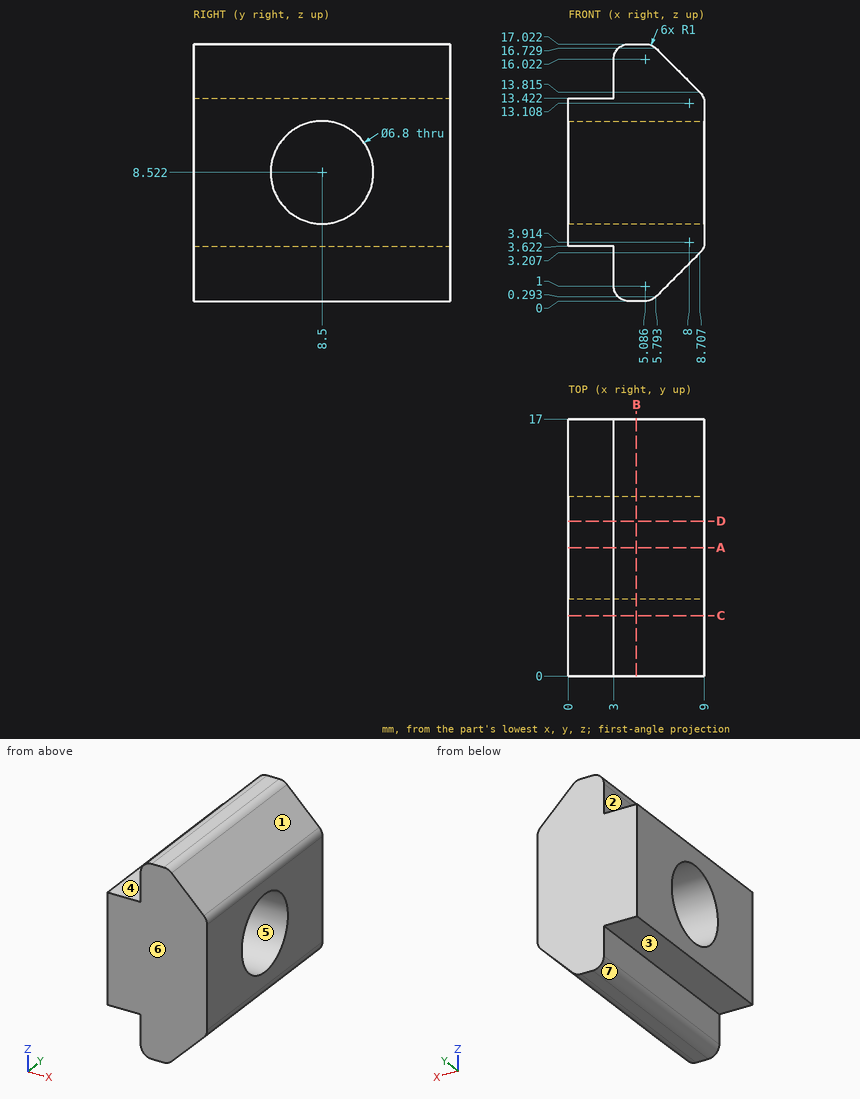
Can you work these out from the drawing? Everything is in mm from the part's minimum corner. A direction names the side the tool comes from. Give positions to 0.01 mm unless a question says otherwise; leave off trailing zeros. Loops run counter-clockwise (first coordinate to the right, second up) from the corner with the lowest first, then second, coordinate; pieces in that order, holes last. Notation, with made-up numbers: M 20,75.25 L 53,75.25 A14 ccw 53,81.25 Z; hole C -6,89.5 d10. An arc over 180 degrees is marked long. Put each result on its own line as item: value. Start each with the question number.
(1) I want a section at D-D on y = 10.25. Please give me the cut outline in (x, z) (1 decimal), then the cut area to 3 significant figures.
(2) For the marked faces 1, 2 and 3, which set-ups out of +Z, -Z, +X, -X, +Y, -Y let a thin tool reach every point of the face, with its end or its side?
(3) If we mould it in two halves opening along Z, with no side actions, what happens to the marked faces 4, 5, 6 and 7? For each: +Z half, -Z half, draft (parallel to the pull), parting line (faces both ways), or undercut.
(4) Will these pins go through, and if not, where does the flat tip stop? pin 1 Ø8 at (y, z) = (9, 8) entering from -X; pin 2 Ø1.3 at (y, z) = (8.5, 14.5) entering from -X; pin 3 Ø2.5 at (x, y) = (2, 4.5) entering from -Z; pin 4 Ø2.5 at (x, y) = (2, 9.5) entering from +Z.
(5) I want a section at B-B on x = 4.5. Please give me the cut outline in (y, z).
(6) I want a section at A-A on y = 8.5. Please give me the cut outline in (x, z) (1 decimal).
(7) I need wall thicknesses on line 1 along Y through (x, z) = (7.25, 5.5); line 2 along Z through (x, y) = (4.5, 6.5); line 3 along Z through (x, y) = (7.5, 6) (1 decimal). Which ranges of each line are inside material? Lowest first, please. Write a range as [from, to].
(8) I want a section at C-C on y = 4. Please give me the cut outline in (x, z) (1 decimal).
Answer block:
1. outline: M 0,3.6 L 3,3.6 L 3,1 A1 ccw 4,0 L 5.1,0 A1 ccw 5.8,0.3 L 8.7,3.2 A1 ccw 9,3.9 L 9,5.6 L 0,5.6 Z; M 0,11.4 L 9,11.4 L 9,13.1 A1 ccw 8.7,13.8 L 5.8,16.7 A1 ccw 5.1,17 L 4,17 A1 ccw 3,16 L 3,13.4 L 0,13.4 Z
1. area: 66.3 mm^2
2. face 1: +Z, +X, +Y, -Y
2. face 2: +Z, -X, +Y, -Y
2. face 3: -Z, -X, +Y, -Y
3. face 4: +Z half
3. face 5: undercut
3. face 6: draft
3. face 7: -Z half
4. pin 1: x = 0
4. pin 2: x = 3
4. pin 3: z = 0.34
4. pin 4: z = 16.68
5. outline: M 0,0 L 17,0 L 17,17.02 L 0,17.02 Z; hole C 8.5,8.52 d6.8
6. outline: M 0,3.6 L 3,3.6 L 3,1 A1 ccw 4,0 L 5.1,0 A1 ccw 5.8,0.3 L 8.7,3.2 A1 ccw 9,3.9 L 9,5.1 L 0,5.1 Z; M 0,11.9 L 9,11.9 L 9,13.1 A1 ccw 8.7,13.8 L 5.8,16.7 A1 ccw 5.1,17 L 4,17 A1 ccw 3,16 L 3,13.4 L 0,13.4 Z
7. line 1: [0, 6.94], [10.06, 17]
7. line 2: [0, 5.77], [11.27, 17.02]
7. line 3: [2, 6.2], [10.8, 15]
8. outline: M 0,3.6 L 3,3.6 L 3,1 A1 ccw 4,0 L 5.1,0 A1 ccw 5.8,0.3 L 8.7,3.2 A1 ccw 9,3.9 L 9,13.1 A1 ccw 8.7,13.8 L 5.8,16.7 A1 ccw 5.1,17 L 4,17 A1 ccw 3,16 L 3,13.4 L 0,13.4 Z
